Verification items for this drawing (mm, ordinates from the low corner). A direction names the side the tool comes from. Round coordinates to 2 decimals unless told otherwise and drop trailing zeros. Order: outer loops, then holes, each group sorted by start corner. A loop starts at its lowest first (then second) coordinate and runs counter-clockwise, first axis right, second up. Notation, with made-up numbers: (3, 18) -> (16, 18) arc R14 ccw to (16, 39) -> close; hole circle Ø3 at (-32.75, -3). An arc over 180 degrees is marked (long way). Return JSON: item names as keys, results as strings. Group by question number.
Item 1: Access from +Z, -Z, +X, -X, +Y, -Y to the whole of each face (thin tool, end or side, straight path). Record for the marked faces 5, 6 and 7.
Item 2: Depth check by flat-ended pin: pin 1 Ø1.8 at (x, z) = (48.5, 1.5) entering from -Y; pin 2 Ø3 at (x, z) = (2.5, 4) entering from +Y; pin 3 Ø1.8 at (y, z) = (102.5, 3.5) entering from +X. Enter the tip coordinate at first touch or a pass-through.
Item 3: Sectioned sample at A-A on y = 99.5. Record the cut outline in (x, z), plus the area to 3 significant figures.
Item 4: Scan lines: probe 1 along Y at (x, z) = (49, 4.9); probe 2 along X at (y, z) = (97, 0.5). Record each from-to range of solid material in increasing order. Write a range as from..to.
Item 5: Draft check along Y on the marked faces 1, 2, 3 and 4. Enter one of: pulls with the +Y half, pulls with the -Y half, needs draft (parallel to the pull), parting line crosses it, or undercut.
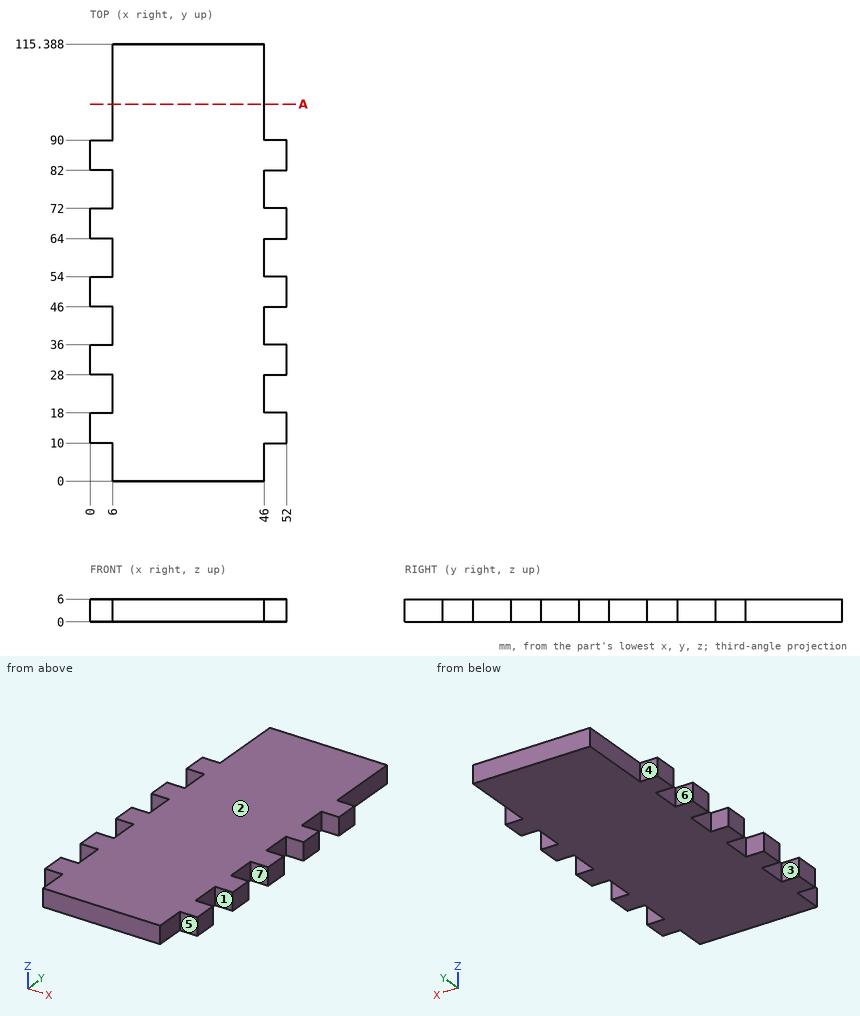
Recorded:
{
 "1": {"face 5": "+Z, -Z, +X, -Y", "face 6": "+Z, -Z, -X", "face 7": "+Z, -Z, +X"},
 "2": {"pin 1": "y = 10", "pin 2": "y = 90", "pin 3": "x = 46"},
 "3": {"outline": "(6, 0) -> (46, 0) -> (46, 6) -> (6, 6) -> close", "area": "240 mm²"},
 "4": {"probe 1": "10..18, 28..36, 46..54, 64..72, 82..90", "probe 2": "6..46"},
 "5": {"face 1": "undercut", "face 2": "needs draft", "face 3": "undercut", "face 4": "pulls with the +Y half"}
}
